Answer from the drawing. Dimensions are ordinates in mm from the lowest x, y and z of the part. A direction names the side the tool comes from. Coordinates: 2 decimals unless noted, no trailing zeros. Write each loop counter-clockwise with the first axis right and the second up, starting at its lowest first coordinate (ties: lowest second). Pieces come first, ordered by that corner, then holes. Notation, with made-up numbers: (-11, 2.5) -> (25, 2.5) arc R29 ccw to (25, 27.5) -> close; hole circle Ø2 at (2.5, 30). An arc over 180 degrees is marked (long way). Answer as a JSON object with one key per item and string values. Group by question number.
(1) For a pull along Y with two mould halves and no side action, classify the marked faces 4 and 5 as +Y half, -Y half, draft (parallel to the pull), parting line (faces both ways), or undercut.
(2) Find section B-B (y = 17). Give the vertices of the cut face in (x, z), then the cut area to 4 significant figures.
(3) Find section C-C (x = 10). Give the vertices of the cut face in (y, z), then the cut area to 4 significant figures.
(4) Find section D-D (z = 24). Give the vertices of the cut face in (x, y).
(5) Straight lines are drawn through the part: L1, parallel to Y at x = 10, z = 16; L2, parallel to Z at x = 6.5, y = 21.25; L3, parallel to X at y = 9.25, z = 13. For each, find the intervals that lie inside material, in ascending order.
(6) Flat-ended cylindrical pins translate along their axes: P1, Ø0.9, axis at x = 10, y = 5.5, coming from the -Z side; P2, Ø0.9, axis at y = 29, z = 30.5, coming from the +X side; P3, Ø4.5, axis at y = 4, z = 4, coming from the +X side; P4, Ø2.5, axis at x = 10, y = 17, coming from the -Z side. Find the tip coordinate at first contact, or state that the pin passes through.
(7) Find section A-A (z = 4). Give the vertices of the cut face in (x, y), then the cut area to 3 significant figures.
(8) Which of the six approach directions +Z, -Z, +X, -X, +Y, -Y give full straight-line access (tool end or side, diameter ignored) to the marked faces 1, 2 and 3?
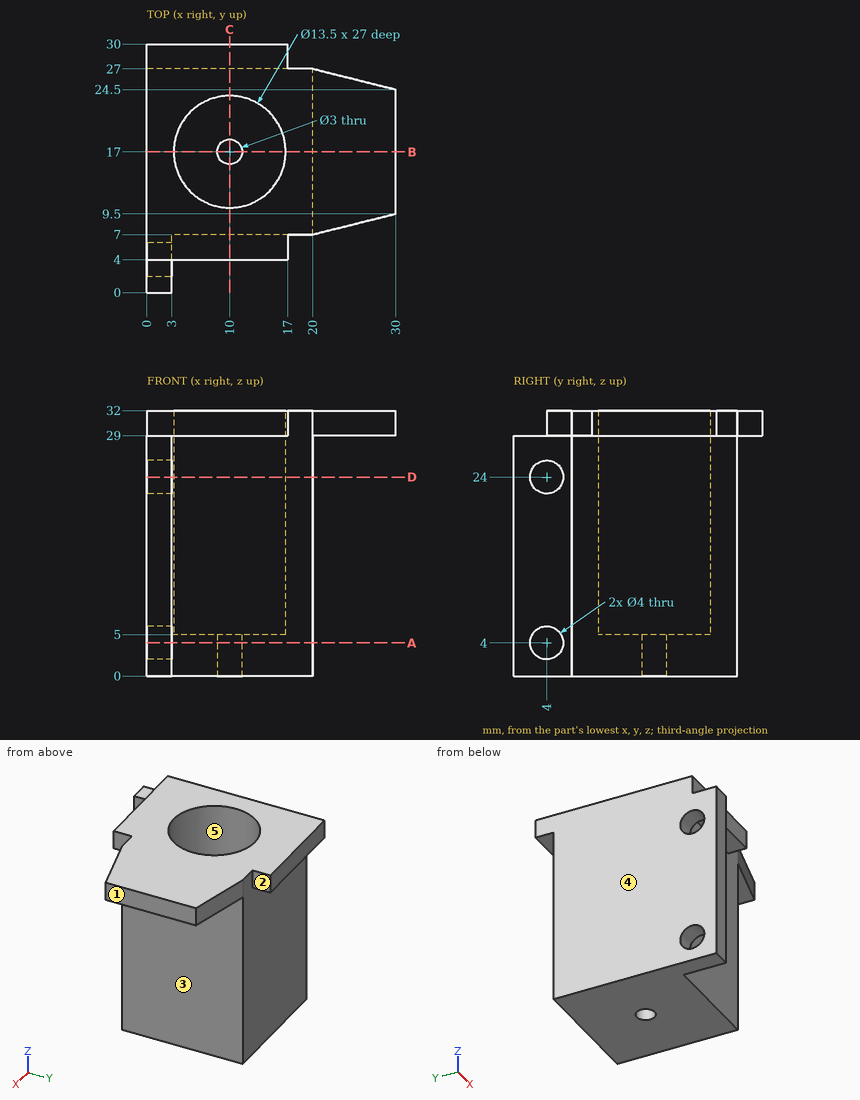
Results below:
{
 "1": {"face 4": "draft", "face 5": "undercut"},
 "2": {"outline": "(0, 0) -> (8.5, 0) -> (8.5, 5) -> (3.25, 5) -> (3.25, 32) -> (0, 32) -> close; (11.5, 0) -> (20, 0) -> (20, 29) -> (30, 29) -> (30, 32) -> (16.75, 32) -> (16.75, 5) -> (11.5, 5) -> close", "area": "290.5 mm2"},
 "3": {"outline": "(4, 29) -> (7, 29) -> (7, 0) -> (15.5, 0) -> (15.5, 5) -> (10.25, 5) -> (10.25, 32) -> (4, 32) -> close; (18.5, 0) -> (27, 0) -> (27, 29) -> (30, 29) -> (30, 32) -> (23.75, 32) -> (23.75, 5) -> (18.5, 5) -> close", "area": "278.5 mm2"},
 "4": {"outline": "(0, 0) -> (3, 0) -> (3, 2) -> (0, 2) -> close; (0, 6) -> (3, 6) -> (3, 7) -> (20, 7) -> (20, 27) -> (0, 27) -> close; hole circle Ø13.5 at (10, 17)"},
 "5": {"L1": "y = 7 to 10.25, 23.75 to 27", "L2": "z = 0 to 5", "L3": "x = 0 to 20"},
 "6": {"P1": "stops at z = 29", "P2": "stops at x = 17", "P3": "stops at x = 3", "P4": "passes through"},
 "7": {"outline": "(0, 0) -> (3, 0) -> (3, 2) -> (0, 2) -> close; (0, 6) -> (3, 6) -> (3, 7) -> (20, 7) -> (20, 27) -> (0, 27) -> close; hole circle Ø3 at (10, 17)", "area": "402 mm2"},
 "8": {"face 1": "+Z, -Z, +X, +Y, -Y", "face 2": "+Z, -Z, +X, +Y", "face 3": "-Z, +X, +Y, -Y"}
}
